The figure shows three views and two pictorial views of one solid part (mm, origin at its lowest corner). Answer the questions. Coordinates: 2 decimals unless noted, no trailing zeros. Write each loop counter-clockwise with the first axis right and the second up, starting at its lowest first coordinate (ties: lowest second). Pieces come first, ordered by that corner, then holes.
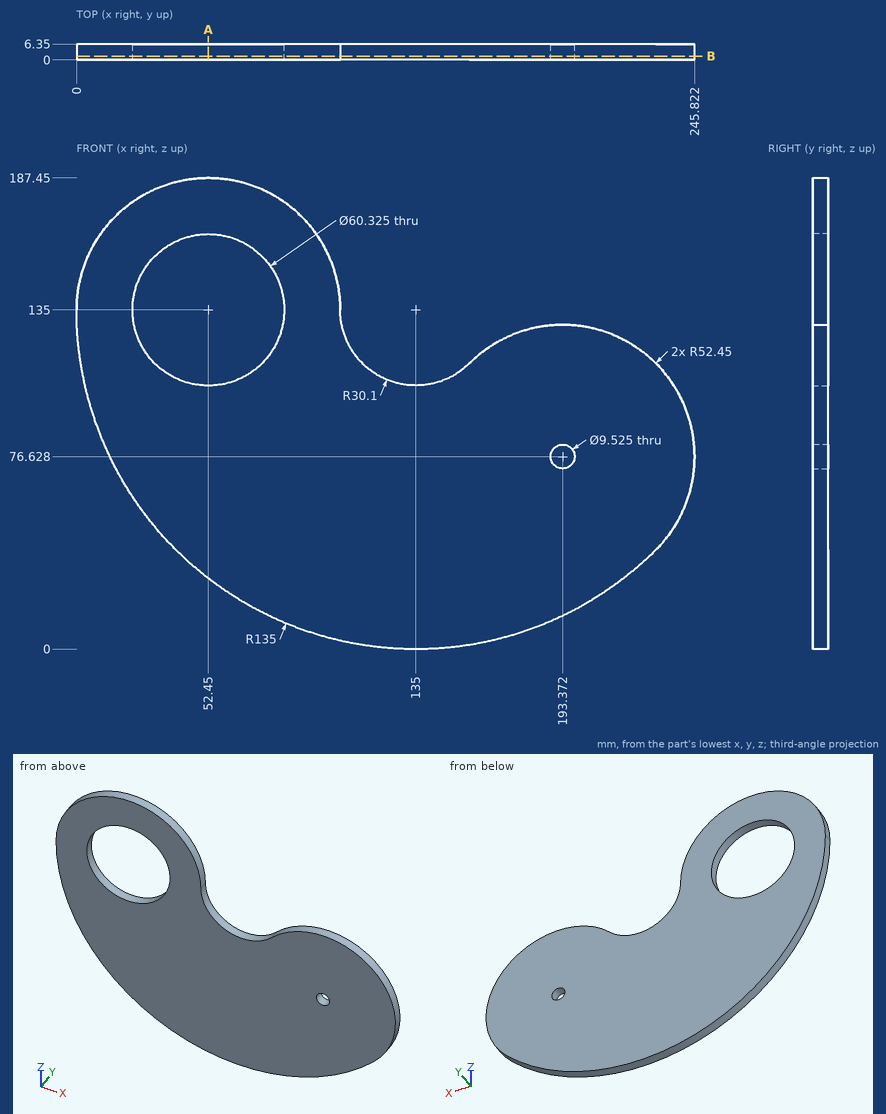
Item 1: Find the intervals of material crossed by probe 1 along X at (y, z) = (2.25, 135); probe 2 along X at (y, z) = (6, 114.5) (1 decimal); probe 3 along X at (y, z) = (2, 148), in increasing order.
Item 2: Given pin 1 (1.5 mm diameter, centred on y = 2.5, z = 96.5, fed in from -X) (1 decimal); pin 2 (1 mm diameter, centred on y = 5.5, z = 36, fed in from -X); pin 3 (1 mm diameter, centred on x = 198.5, y = 5, fed in from +Z), each flat-ended and moving along its own axis, determine where each tip first touches the part or whether it passes through.
Item 3: The part is cut by section A-A (x = 52.45). Give the vertices of the cut face in (y, z), and give its area (3 significant figures).
Item 4: The part is cut by section B-B (y = 1.5). State how many separate pieces and enclosed holes the cut face has, and give its area (3 significant figures).
Answer:
1. probe 1: x = 0 to 22.29, 82.61 to 104.9
1. probe 2: x = 1.6 to 30.3, 74.6 to 113, 157.1 to 229.7
1. probe 3: x = 1.64 to 25.23, 79.67 to 103.26
2. pin 1: stops at x = 5.4
2. pin 2: stops at x = 42.68
2. pin 3: stops at z = 128.87
3. outline: (0, 28.18) - (6.35, 28.18) - (6.35, 104.84) - (0, 104.84) - close; (0, 165.16) - (6.35, 165.16) - (6.35, 187.45) - (0, 187.45) - close
3. area: 628 mm2
4. separate pieces: 1
4. enclosed holes: 2
4. area: 26,100 mm2
